For this review, take the finished solid that the model builds, in its own axes (mm). Face numbers are marked on the shaded views. A direction names the side the tool comes from. Give positions to 0.01 mm unless a question says otherwise; leave off trailing zeros. Write each loop counter-clockwise with the first axis right and the second up, starting at its lowest first coordinate (ties: lowest second). Pieces come first, ordered by that corner, then holes.
Q1. Insertion check: P1, Ø0.6, axis at x = 1.5, z = -0.5, coming from the -Y side; P2, Ø2, axis at x = -3.5, y = -0.5, coming from the -Z side; P3, Ø0.6, axis at x = 0.5, z = -1, coming from the +Y side; P4, Ø1, axis at x = -3.5, y = 1.5, coming from the +Z side. Each pin has a flat end and moves straight along its axis. Give the tip position at first contact, or say it passes through.
Q2. We need section C-C (z = 2.75). Write out the cut boundary in (x, y), then the cut area to 3 significant figures.
Q3. We need section D-D (x = 0.25). Write out the cut boundary in (y, z).
Q4. Mouldability with a two-part tool opening along Y and no side actions: class the marked faces 6, 7 and 8 as released by +Y, released by -Y, zero draft, split by the parting line, or undercut.
Q5. We need section B-B (x = -3.5). Write out the cut boundary in (y, z), then the cut area to 3 significant figures.
Q6. For line 1 (Y direction, x = 1.5, z = 6); line 2 (Y direction, x = -0.5, z = -0.25); line 3 (Z direction, x = -3.5, y = -3.25), list the stretches that pass through material, from the lowest coordinate up.
Q7. Machinability: for the marked faces 1, 2, 3, 4 and 5, which of the approach directions +Z, -Z, +X, -X, +Y, -Y give a long, thin tool a straight path to every point of the face, cutting with its end or side? Answer none if there is none.
Q8. We need section A-A (z = 6.25). Write out the cut boundary in (x, y).
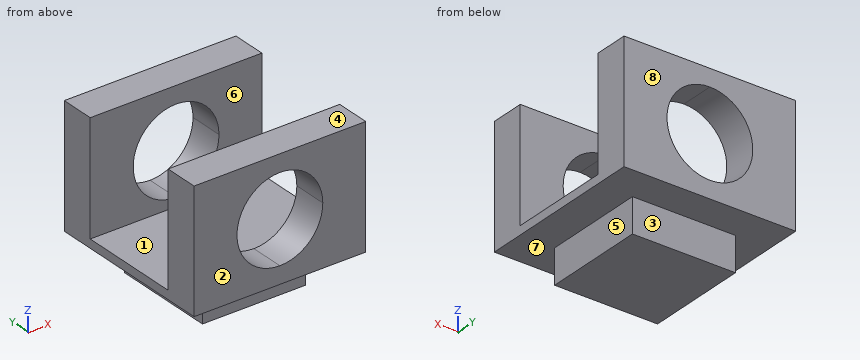
```python
from build123d import *

# Parameters (mm, degrees)
F0_W     = 6
F0_H     = 6
F1_DEPTH = 2
F0_W_2   = 2
F2_DEPTH = 0.5
F4_DEPTH = 10
F5_W     = 10
F5_H     = 6
F6_DEPTH = 6.5


with BuildPart() as f1:
    # F0 (on Top) → F1 (new body)
    with BuildSketch(Plane.XY):
        Rectangle(F0_W, F0_H)
    extrude(amount=-F1_DEPTH)

    # F0 (on Top) → F2 (join)
    with BuildSketch(Plane.XY):
        Polygon((5, 3), (5, 5), (-5, 5), (-5, 3), (-3, 3), (3, 3), align=None)
        Rectangle(F0_W, F0_H)
        with Locations((-4, 0)):
            Rectangle(F0_W_2, F0_H)
        Polygon((5, -5), (5, -3), (3, -3), (-3, -3), (-5, -3), (-5, -5), align=None)
        with Locations((4, 0)):
            Rectangle(F0_W_2, F0_H)
    extrude(amount=F2_DEPTH)

    # F3 (on face) → F4 (join)
    with BuildSketch(Plane.XZ.offset(5)):
        with BuildLine():
            Line((0, 1), (0, 0.5))
            Line((0, 0.5), (5, 0.5))
            Line((5, 0.5), (5, 7))
            Line((5, 7), (0, 7))
            Line((0, 7), (0, 6))
            ThreePointArc((0, 6), (1.767767, 5.267767), (2.5, 3.5))
            ThreePointArc((2.5, 3.5), (1.767767, 1.732233), (0, 1))
        make_face()
        with BuildLine():
            Line((-5, 7), (-5, 0.5))
            Line((-5, 0.5), (0, 0.5))
            Line((0, 0.5), (0, 1))
            ThreePointArc((0, 1), (-2.5, 3.5), (0, 6))
            Line((0, 6), (0, 7))
            Line((0, 7), (-5, 7))
        make_face()
    extrude(amount=-F4_DEPTH)

    # F5 (on face) → F6 (cut)
    with BuildSketch(Plane.XY.offset(7)):
        Rectangle(F5_W, F5_H)
    extrude(amount=-F6_DEPTH, mode=Mode.SUBTRACT)


solid = f1.part
```
Computed:
1. P1: stops at y = -3
1. P2: stops at z = -2
1. P3: stops at y = 3
1. P4: stops at z = 0.5
2. outline: (-5, -5) - (-2.38, -5) - (-2.38, -3) - (-5, -3) - close; (-5, 3) - (-2.38, 3) - (-2.38, 5) - (-5, 5) - close; (2.38, -5) - (5, -5) - (5, -3) - (2.38, -3) - close; (2.38, 3) - (5, 3) - (5, 5) - (2.38, 5) - close
2. area: 20.9 mm2
3. outline: (-5, 0) - (-3, 0) - (-3, -2) - (3, -2) - (3, 0) - (5, 0) - (5, 1.01) - (3, 1.01) - (3, 0.5) - (-3, 0.5) - (-3, 1.01) - (-5, 1.01) - close; (-5, 5.99) - (-3, 5.99) - (-3, 7) - (-5, 7) - close; (3, 5.99) - (5, 5.99) - (5, 7) - (3, 7) - close
4. face 6: undercut
4. face 7: zero draft
4. face 8: released by +Y
5. outline: (-5, 0) - (5, 0) - (5, 7) - (3, 7) - (3, 0.5) - (-3, 0.5) - (-3, 7) - (-5, 7) - close
5. area: 31.0 mm2
6. line 1: y = -5 to -3, 3 to 5
6. line 2: y = -3 to 3
6. line 3: z = 0 to 7
7. face 1: +Z, +X, -X
7. face 2: +Z, -Z, +X, -X, -Y
7. face 3: -Z, +X, -X, +Y
7. face 4: +Z, +X, -X, +Y, -Y
7. face 5: -Z, +X, +Y, -Y
8. outline: (-5, -5) - (5, -5) - (5, -3) - (-5, -3) - close; (-5, 3) - (5, 3) - (5, 5) - (-5, 5) - close
